CAD build for the part. Positions are in the model's coordinates, mm. A direction names the side the tool comes from. Give positions to 0.01 mm unless a question says otherwise; leave off trailing zeros. Order: outer loops, then holes, each group sorted by start corner. A loop starts at its lowest first (then second) coordinate and runs counter-clockwise, first axis right, second up.
Item 1: Two-plate mould, pull along X, no slides. Class faces 3 (the flat face through (0, -28, 2)), 4 (the cylindrical face through (52.99, -53.15, 2.54)), 5 (the flat face through (28, 0, 2)), 6 (the flat face through (22.535, -33.669, 2.535)): released by +X, released by -X, zero draft, split by the parting line, or undercut.
Item 2: Band-saw the part on B-B on y = -51.5. Give the cut face in (x, z), plus the area to 3 significant figures.
Item 3: Band-saw the part on A-A on z = 2.05. Count the separate pieces of the cut face and the enclosed holes in it, plus the area to 3 significant figures.
Item 4: Wall check: L1, parallel to Y at x = 14, z = 3.85; L2, parallel to X at y = -28, z = 0.9; L3, parallel to Y at x = 9.5, z = 3.5. Give the ranges that are in metal, low to high.
Item 5: Flat gauge pin, fed straight in: P1, Ø5, axis at x = 9.5, y = -30.5, coming from the +Z side. Where does the tip first touch, or does it go through?
Item 6: Which spindle directions (+Z, -Z, +X, -X, +Y, -Y) get a long thin tool onto all of the face, cutting with end or side? Do faces 1 (the flat face through (45, -48, 3)), 2 (the flat face through (34, -34, 5)). Say none if no direction does.
```python
from build123d import *

# Parameters (mm, degrees)
SKETCH_1_W          = 56
SKETCH_1_H          = 56
SKETCH_1_R          = 2.1
EXTRUDE_1_DEPTH     = 5
FILLET_1_R          = 10
CUT_EXTRUDE_1_DEPTH = 16
CUT_EXTRUDE_2_DEPTH = 16


with BuildPart() as part:
    # 草图1 → 凸台-拉伸1 (new body)
    with BuildSketch(Plane.XY):
        with Locations((28, -28)):
            Rectangle(SKETCH_1_W, SKETCH_1_H)
        with Locations((36.625, -13.061061785)):
            Circle(SKETCH_1_R, mode=Mode.SUBTRACT)
        with Locations((19.375, -13.061061785)):
            Circle(SKETCH_1_R, mode=Mode.SUBTRACT)
        with Locations((36.625, -42.938938215)):
            Circle(SKETCH_1_R, mode=Mode.SUBTRACT)
        with Locations((19.375, -42.938938215)):
            Circle(SKETCH_1_R, mode=Mode.SUBTRACT)
    extrude(amount=EXTRUDE_1_DEPTH)

    # 圆角1
    fillet_1_edges = [part.edges().sort_by_distance(p)[0] for p in [
        (56, -56, 2.5),
        (0, -56, 2.5),
        (0, 0, 2.5),
        (56, 0, 2.5),
    ]]
    fillet(fillet_1_edges, radius=FILLET_1_R)

    # 草图2 → 切除-拉伸1 (cut)
    with BuildSketch(Plane.XY.offset(5)):
        with BuildLine():
            Line((47.15, -8), (43.05, -8))
            ThreePointArc((43.05, -8), (42.757106781, -8.707106781), (42.05, -9))
            Line((42.05, -9), (42.05, -47))
            ThreePointArc((42.05, -47), (42.757106781, -47.292893219), (43.05, -48))
            Line((43.05, -48), (47.15, -48))
            ThreePointArc((47.15, -48), (47.442893219, -47.292893219), (48.15, -47))
            Line((48.15, -47), (48.15, -9))
            ThreePointArc((48.15, -9), (47.442893219, -8.707106781), (47.15, -8))
        make_face()
        with BuildLine():
            ThreePointArc((43.05, -8), (42.757106781, -7.292893219), (42.05, -7))
            Line((42.05, -7), (42.05, -8))
            Line((42.05, -8), (43.05, -8))
        make_face()
        with BuildLine():
            Line((43.05, -8), (42.05, -8))
            Line((42.05, -8), (42.05, -9))
            ThreePointArc((42.05, -9), (42.757106781, -8.707106781), (43.05, -8))
        make_face()
        with BuildLine():
            Line((42.05, -8), (42.05, -7))
            ThreePointArc((42.05, -7), (41.05, -8), (42.05, -9))
            Line((42.05, -9), (42.05, -8))
        make_face()
        with BuildLine():
            ThreePointArc((49.15, -8), (48.15, -7), (47.15, -8))
            Line((47.15, -8), (48.15, -8))
            Line((48.15, -8), (48.15, -9))
            ThreePointArc((48.15, -9), (48.857106781, -8.707106781), (49.15, -8))
        make_face()
        with BuildLine():
            Line((48.15, -8), (47.15, -8))
            ThreePointArc((47.15, -8), (47.442893219, -8.707106781), (48.15, -9))
            Line((48.15, -9), (48.15, -8))
        make_face()
        with BuildLine():
            ThreePointArc((49.15, -48), (48.857106781, -47.292893219), (48.15, -47))
            Line((48.15, -47), (48.15, -48))
            Line((48.15, -48), (47.15, -48))
            ThreePointArc((47.15, -48), (48.15, -49), (49.15, -48))
        make_face()
        with BuildLine():
            Line((48.15, -48), (48.15, -47))
            ThreePointArc((48.15, -47), (47.442893219, -47.292893219), (47.15, -48))
            Line((47.15, -48), (48.15, -48))
        make_face()
        with BuildLine():
            ThreePointArc((43.05, -48), (42.757106781, -47.292893219), (42.05, -47))
            Line((42.05, -47), (42.05, -48))
            Line((42.05, -48), (43.05, -48))
        make_face()
        with BuildLine():
            Line((43.05, -48), (42.05, -48))
            Line((42.05, -48), (42.05, -49))
            ThreePointArc((42.05, -49), (42.757106781, -48.707106781), (43.05, -48))
        make_face()
        with BuildLine():
            Line((42.05, -48), (42.05, -47))
            ThreePointArc((42.05, -47), (41.05, -48), (42.05, -49))
            Line((42.05, -49), (42.05, -48))
        make_face()
        with BuildLine():
            Line((13.95, -48), (13.95, -47))
            ThreePointArc((13.95, -47), (13.242893219, -47.292893219), (12.95, -48))
            Line((12.95, -48), (13.95, -48))
        make_face()
        with BuildLine():
            ThreePointArc((12.95, -48), (13.242893219, -48.707106781), (13.95, -49))
            Line((13.95, -49), (13.95, -48))
            Line((13.95, -48), (12.95, -48))
        make_face()
        with BuildLine():
            ThreePointArc((14.95, -48), (14.657106781, -47.292893219), (13.95, -47))
            Line((13.95, -47), (13.95, -48))
            Line((13.95, -48), (13.95, -49))
            ThreePointArc((13.95, -49), (14.657106781, -48.707106781), (14.95, -48))
        make_face()
        with BuildLine():
            ThreePointArc((13.95, -9), (13.242893219, -8.707106781), (12.95, -8))
            Line((12.95, -8), (8.85, -8))
            ThreePointArc((8.85, -8), (8.557106781, -8.707106781), (7.85, -9))
            Line((7.85, -9), (7.85, -47))
            ThreePointArc((7.85, -47), (8.557106781, -47.292893219), (8.85, -48))
            Line((8.85, -48), (12.95, -48))
            ThreePointArc((12.95, -48), (13.242893219, -47.292893219), (13.95, -47))
            Line((13.95, -47), (13.95, -9))
        make_face()
        with BuildLine():
            ThreePointArc((8.85, -48), (8.557106781, -47.292893219), (7.85, -47))
            Line((7.85, -47), (7.85, -48))
            Line((7.85, -48), (8.85, -48))
        make_face()
        with BuildLine():
            Line((7.85, -48), (7.85, -47))
            ThreePointArc((7.85, -47), (7.142893219, -48.707106781), (8.85, -48))
            Line((8.85, -48), (7.85, -48))
        make_face()
        with BuildLine():
            ThreePointArc((7.85, -9), (8.557106781, -8.707106781), (8.85, -8))
            Line((8.85, -8), (7.85, -8))
            Line((7.85, -8), (7.85, -9))
        make_face()
        with BuildLine():
            Line((7.85, -8), (8.85, -8))
            ThreePointArc((8.85, -8), (7.142893219, -7.292893219), (7.85, -9))
            Line((7.85, -9), (7.85, -8))
        make_face()
        with BuildLine():
            ThreePointArc((14.95, -8), (14.657106781, -7.292893219), (13.95, -7))
            Line((13.95, -7), (13.95, -8))
            Line((13.95, -8), (13.95, -9))
            ThreePointArc((13.95, -9), (14.657106781, -8.707106781), (14.95, -8))
        make_face()
        with BuildLine():
            Line((13.95, -8), (13.95, -7))
            ThreePointArc((13.95, -7), (13.242893219, -7.292893219), (12.95, -8))
            Line((12.95, -8), (13.95, -8))
        make_face()
        with BuildLine():
            Line((13.95, -9), (13.95, -8))
            Line((13.95, -8), (12.95, -8))
            ThreePointArc((12.95, -8), (13.242893219, -8.707106781), (13.95, -9))
        make_face()
    extrude(amount=-CUT_EXTRUDE_1_DEPTH, mode=Mode.SUBTRACT)

    # 草图3 → 切除-拉伸2 (cut)
    with BuildSketch(Plane.XY.offset(5)):
        with BuildLine():
            Line((25.657393572, -18.428258035), (19.499268114, -26.125914857))
            ThreePointArc((19.499268114, -26.125914857), (18.841874542, -28), (19.499268114, -29.874085143))
            Line((19.499268114, -29.874085143), (25.657393572, -37.571741965))
            ThreePointArc((25.657393572, -37.571741965), (28, -38.697656822), (30.342606428, -37.571741965))
            Line((30.342606428, -37.571741965), (36.500731886, -29.874085143))
            ThreePointArc((36.500731886, -29.874085143), (37.158125458, -28), (36.500731886, -26.125914857))
            Line((36.500731886, -26.125914857), (30.342606428, -18.428258035))
            ThreePointArc((30.342606428, -18.428258035), (28, -17.302343178), (25.657393572, -18.428258035))
        make_face()
    extrude(amount=-CUT_EXTRUDE_2_DEPTH, mode=Mode.SUBTRACT)


solid = part.part
```
The answers:
1. face 3: released by -X
1. face 4: released by +X
1. face 5: zero draft
1. face 6: undercut
2. outline: (1.65, 0) - (54.35, 0) - (54.35, 5) - (1.65, 5) - close
2. area: 264 mm2
3. separate pieces: 1
3. enclosed holes: 7
3. area: 2,250 mm2
4. L1: y = -56 to -49, -47 to -9, -7 to 0
4. L2: x = 0 to 7.85, 13.95 to 18.84, 37.16 to 42.05, 48.15 to 56
4. L3: y = -55.99 to -48, -8 to -0.01
5. P1: stops at z = 5
6. face 1: +Z, -Z
6. face 2: +Z, +X, -X, +Y, -Y
